Could you check a few things on this model? Use its own coordinates, in mm. A direction names the side the tool comes from. Give positions to 0.01 mm unless a question says otherwise; leave off trailing zeros. Write each loop counter-clockwise with the first axis right and the second up, starting at its lowest first coordinate (ties: lowest second). Pieces come first, ordered by that corner, then holes. Notation, with made-up numbers: (-10.75, -26) - (36.25, -26) arc R25 ccw to (36.25, -11) - close; hole circle Ø7 at (-8.75, 78). An arc over 180 degrees is marked (long way). Write item = value, one per line.
Autodesk Inventor part; units mm, degrees
ref_plane "YZ Plane" through (0, 0, 0) normal (1, 0, 0) x (0, 1, 0)
ref_plane "XZ Plane" through (0, 0, 0) normal (0, 1, 0) x (-1, 0, 0)
ref_plane "XY Plane" through (0, 0, 0) normal (0, 0, 1) x (1, 0, 0)
sketch "Sketch1" plane through (0, 0, 0) normal (0, 1, 0) x (-1, 0, 0)
  line L0 (-3.75, -25) -> (-3.75, 23)
  line L1 (-1.75, 25) -> (1.75, 25)
  line L2 (3.75, 23) -> (3.75, -25)
  line L3 (3.75, -25) -> (-3.75, -25)
  line L4 (-3.75, -25) -> (3.75, 25) construction
  line L5 (-3.75, 25) -> (3.75, -25) construction
  line L6 (0, 0.8712) -> (0, 20.8712) construction
  line L7 (-1.7, 0.8712) -> (-1.7, 20.8712)
  line L8 (1.7, 20.8712) -> (1.7, 0.8712)
  arc A0 (-1.7, 0.8712) -> (1.7, 0.8712) centre (0, 0.8712) ccw
  arc A1 (1.7, 20.8712) -> (-1.7, 20.8712) centre (0, 20.8712) ccw
  arc A2 (3.75, 23) -> (1.75, 25) centre (1.75, 23) ccw
  arc A3 (-1.75, 25) -> (-3.75, 23) centre (-1.75, 23) ccw
  line L9 (-3.75, -25) -> (12.9085, -8.3415)
  line L10 (12.9085, -8.3415) -> (15.4834, -10.9164)
  line L11 (15.4834, -10.9164) -> (-1.1751, -27.5749)
  line L12 (-1.1751, -27.5749) -> (-3.75, -25)
  arc A4 (3.75, -4.8061) -> (3.75, -20.0848) centre (12.1805, -12.4455) ccw
  point P0 (0, 0)
  point P1 (0, 10.8712)
  point P2 (1.3998, -25)
  point P3 (3.75, -17.5)
  point P4 (2.627, -18.623)
  dimension "d0" = 7.5
  dimension "d1" = 50
  dimension "d2" = 20
  dimension "d3" = 1.7
  dimension "d4" = 2
  dimension "d8" = 45
extrude "Main Arm" add sketch "Sketch1" along normal blind 4 contours L9 A4 L2 L11 L3 | L0 A3 L1 A2 L2 A4 L9 | L9 L2 A4 | L2 L9 L10 L11 picked at (3.6165, -19.0676)
sketch "Pad holder" plane through (-15.4834, 0, -10.9164) normal (-0.7071068, 0, -0.7071068) x (-0.7071068, 0, 0.7071068)
  line L0 (-3.8154, 0) -> (-3.8154, 4)
  circle A0 centre (-3.8154, 2) radius 12.5
  point P0 (-3.2294, 0)
  dimension "d9" = 25
extrude "pad area" add sketch "Pad holder" against normal blind 7
hole "Hole1" at (-12.7855, 2, -13.6143) direction (0.7071068, 0, 0.7071068) diameter 5.0038 depth 7
sketch "Screw position" plane through (-10.5337, 0, -5.9666) normal (0.7071068, 0, 0.7071068) x (0.7071068, 0, -0.7071068)
  line L0 (3.8154, 0) -> (3.8154, 4)
  line L1 (3.8154, 7.4848) -> (8.5654, 4.7424)
  line L2 (8.5654, 4.7424) -> (8.5654, -0.7424)
  line L3 (8.5654, -0.7424) -> (3.8154, -3.4848)
  line L4 (3.8154, -3.4848) -> (-0.9346, -0.7424)
  line L5 (-0.9346, -0.7424) -> (-0.9346, 4.7424)
  line L6 (-0.9346, 4.7424) -> (3.8154, 7.4848)
  point P0 (3.2294, 0)
  point P1 (3.8154, 2)
  dimension "d21" = 9.5
extrude "Extrusion3" cut sketch "Screw position" against normal blind 4
fillet "Fillet1" radius 6 3 edges at (-1.3998, 2, -25) (3.75, 2, -25) (-3.75, 2, -4.8061)
fillet "Fillet2" radius 2 1 edges at (-1.1744, 2, -15.326)
properties part number "arm"
1. If we section it at D-D, the plane y = -4.5: Please give me the cut outline in (x, z).
Filled sheet:
outline = (-20.34, -6.06) - (-6.49, -19.91) arc R6 ccw to (-5.05, -20.97) - (-0.29, -16.21) - (-15.39, -1.11) - close
2. Which directions (+Z, -Z, +X, -X, +Y, -Y) give clear straight access to the entire face, cutting with the end or side of a thin tool? Please do faces 5 (the face through (-14, -0.6, -12.4)), 6 (the face through (-5.872, 2.038, -13.418)), 7 (the face through (0.04, 1.97, 22.57)), 8 (the face through (-10.934, 6.094, -8.357)).
Filled sheet:
face_5 = -Z, -X, +Y, -Y
face_6 = +Z
face_7 = +Y, -Y
face_8 = none
3. If we section it at B-B, the plane y = 6.25: Please give me the cut outline in (x, z).
Filled sheet:
outline = (-21.1, -5.3) - (-6.49, -19.91) arc R6 ccw to (-3.96, -21.42) - (0.48, -16.98) - (-6.32, -10.18) - (-9.15, -13.01) - (-12.18, -9.98) - (-9.35, -7.15) - (-16.15, -0.35) - close
4. Thinking about a two-plate mould opening in X: for faces 1 (the face through (-1.7, 2, 11)), 2 (the face through (3.75, 2, 3)), 3 (the face through (-3.497, 1.972, -4.488)), 4 (the face through (-3.15, 1.97, 24.43)), which applies, pulls with the +X half, pulls with the -X half, needs draft (parallel to the pull), parting line crosses it, or undercut?
Filled sheet:
face_1 = undercut
face_2 = pulls with the +X half
face_3 = undercut
face_4 = pulls with the -X half
5. For pin 1 (4.5 mm diameter, centred on y = 2.5, z = 12, fed in from -X); pin 2 (6 mm diameter, centred on x = 0.5, z = 1.5, fed in from +Y); pin 3 (1.5 mm diameter, centred on x = 0.5, z = -10.5, fed in from -Y), each with a flat end and sliding along its axis, tell me the tip position at first contact or that it passes through.
Filled sheet:
pin_1 = -3.75
pin_2 = 4
pin_3 = 0
6. I need wall thicknesses on line 1 (X direction, y = 3.5, z = 3.5); line 2 (Y direction, x = -7, z = -14); line 3 (Y direction, x = -16.75, z = -5). Which ranges of each line are inside material? Lowest first, please.
Filled sheet:
line_1 = -3.75 to -1.7, 1.7 to 3.75
line_2 = -9.71 to -0.97, 4.97 to 13.71
line_3 = -6.78 to 10.78
7. If we section it at C-C, the plane z = 21.5: Please give me the cut outline in (x, y).
Filled sheet:
outline = (-3.75, 0) - (-1.58, 0) - (-1.58, 4) - (-3.75, 4) - close; (1.58, 0) - (3.75, 0) - (3.75, 4) - (1.58, 4) - close
8. If we section it at A-A, the plane z = 14: Please give me the cut outline in (x, y).
Filled sheet:
outline = (-3.75, 0) - (-1.7, 0) - (-1.7, 4) - (-3.75, 4) - close; (1.7, 0) - (3.75, 0) - (3.75, 4) - (1.7, 4) - close
